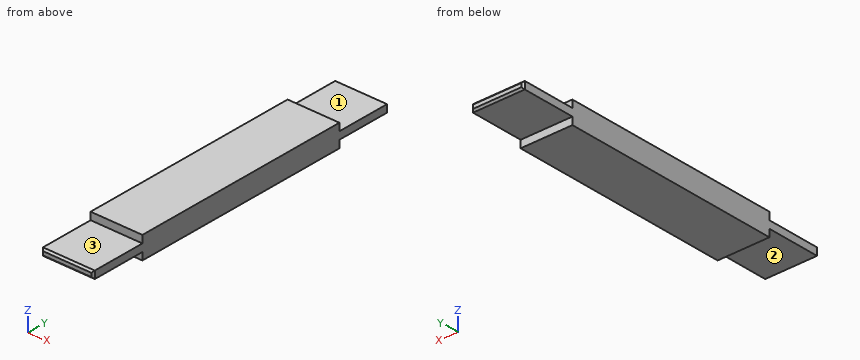
```python
from build123d import *

# Parameters (mm, degrees)
F0_W     = 88.9
F0_H     = 38.1
F1_DEPTH = 190.5
F2_W     = 88.9
F2_H     = 12.7
F3_DEPTH = 95.25
F4_SIZE  = 3.175


with BuildPart() as f1:
    # F0 (on Front) → F1 (new body)
    with BuildSketch(Plane.XZ):
        with Locations((44.45, 19.05)):
            Rectangle(F0_W, F0_H)
    extrude(amount=F1_DEPTH)

    # F2 (on face) → F3 (join)
    with BuildSketch(Plane.XZ.offset(190.5)):
        with Locations((44.45, 19.05)):
            Rectangle(F2_W, F2_H)
    extrude(amount=F3_DEPTH)

    # F4
    f4_edges = [f1.edges().sort_by_distance(p)[0] for p in [
        (44.45, -285.75, 25.4),
        (0, -285.75, 19.05),
        (44.45, -285.75, 12.7),
        (88.9, -285.75, 19.05),
    ]]
    chamfer(f4_edges, length=F4_SIZE)

    # F5: F1 across face


with BuildPart() as f1_1:
    add(f1.part)
    add(f1.part.mirror(Plane(origin=(44.45, 0, 19.05), x_dir=(1, 0, 0), z_dir=(0, 1, 0))))


solid = f1_1.part
```
Verification items for the finished model (mm, model axes). Face numbers are marked on the shaded views. A direction names the side the tool comes from. Coordinates: 2 decimals unless noted, no trailing zeros. Loops run counter-clockwise (first coordinate to the right, second up) from the corner with the lowest first, then second, coordinate; pieces in that order, holes last. Notation, with made-up numbers: (-24, 83) -> (19, 83) arc R11 cw to (19, 89) -> close; hole circle Ø3 at (84.25, 41.5). An arc over 180 degrees is marked (long way). Put each result on its own line as item: value.
1. Gauge pin test, flat ends, axial feed: P1, Ø12, axis at x = 34, z = 34.5, coming from the -Y side; P2, Ø4, axis at x = 29.5, z = 32.5, coming from the +Y side; P3, Ø5, axis at x = 77, y = 218.5, coming from the -Z side; P4, Ø3, axis at x = 28.5, y = -17, coming from the -Z side. Record the tip position at first contact, or that the pin passes through.
Result set:
P1: stops at y = -190.5
P2: stops at y = 190.5
P3: stops at z = 12.7
P4: stops at z = 0
2. Tool access check on the marked faces 1, 2 and 3. Record the directions out of +Z, -Z, +X, -X, +Y, -Y that give a thin tool (end or side, any length) a straight path to the whole face; none if there is none.
Result set:
face 1: +Z, +X, -X, +Y
face 2: -Z, +X, -X, -Y
face 3: +Z, +X, -X, -Y
3. Section check A-A, the plane x = 23. Record the boundary of the cut face in (y, z) (3 decimals).
Result set:
outline: (-285.75, 15.875) -> (-282.575, 12.7) -> (-190.5, 12.7) -> (-190.5, 0) -> (190.5, 0) -> (190.5, 12.7) -> (282.575, 12.7) -> (285.75, 15.875) -> (285.75, 22.225) -> (282.575, 25.4) -> (190.5, 25.4) -> (190.5, 38.1) -> (-190.5, 38.1) -> (-190.5, 25.4) -> (-282.575, 25.4) -> (-285.75, 22.225) -> close
4. Thickness scan on line 1 (Y direction, x = 66, z = 30); line 2 (Z direction, x = 77.5, y = 232); line 3 (Y direction, x = 15, z = 13.5) (3 decimals). Record the ranges inside material, lowest first.
Result set:
line 1: y = -190.5 to 190.5
line 2: z = 12.7 to 25.4
line 3: y = -283.375 to 283.375
5. Section check B-B, the plane y = -199. Record the boundary of the cut face in (x, z), then the cut area to 3 significant figures.
Result set:
outline: (0, 12.7) -> (88.9, 12.7) -> (88.9, 25.4) -> (0, 25.4) -> close
area: 1,130 mm^2
6. Section check C-C, the plane z = 33. Record the boundary of the cut face in (x, y), then the cut area to 3 significant figures.
Result set:
outline: (0, -190.5) -> (88.9, -190.5) -> (88.9, 190.5) -> (0, 190.5) -> close
area: 33,900 mm^2
